Model file for the job. Use its own axes, mm. A direction names the side the tool comes from. Give positions to 0.01 mm unless a question says otherwise; leave off trailing zeros. Loops run counter-clockwise (first coordinate to the right, second up) from the corner with the lowest first, then second, coordinate; pieces in that order, holes last. Notation, with made-up numbers: (24.5, 25) - (28.5, 25) arc R16 cw to (28.5, 55) - close; hole circle Ø2 at (76, 51.25). An arc over 180 degrees is marked (long way). Use a Markdown table: item, result.
from build123d import *

# Parameters (mm, degrees)
F0_R        = 1.6
F1_DEPTH    = 1.5
F2_DEPTH    = 3.5
F3_T1_DEPTH = 1.5
F4_R        = 5


# Not quite as in the source:
# - a fillet or chamfer that OpenCascade refuses, or shapes differently, is made with other operations: its cross-section is extruded or revolved along the edge and cut away or added
# - a feature names something its author has since deleted; it is built from what else it names


with BuildPart() as f1:
    # F0 (on Top) → F1 (new body)
    with BuildSketch(Plane.XY):
        with BuildLine():
            Line((-18.9040250808, 5.7581766099), (-18.9040250808, 11.7581766099))
            Line((-18.9040250808, 11.7581766099), (-23.6040250808, 11.7581766099))
            Line((-23.6040250808, 11.7581766099), (-24.9040250808, 11.7581766099))
            Line((-24.9040250808, 11.7581766099), (-24.9040250808, -15.541421883))
            ThreePointArc((-24.9040250808, -15.541421883), (-22.6536235737, -17.7918233901), (-24.9040250808, -20.0422248973))
            Line((-24.9040250808, -20.0422248973), (-24.9040250808, -24.3918233901))
            ThreePointArc((-24.9040250808, -24.3918233901), (-21.9040250808, -21.3918233901), (-18.9040250808, -24.3918233901))
            Line((-18.9040250808, -24.3918233901), (-18.9040250808, -22.1418233901))
            Line((-18.9040250808, -22.1418233901), (-18.9040250808, -16.1418233901))
            Line((-18.9040250808, -16.1418233901), (-18.9040250808, 5.7581766099))
        make_face()
        with BuildLine():
            ThreePointArc((33.3459749192, 8.7581766099), (28.2246545756, 6.6368562663), (30.3459749192, 11.7581766099))
            Line((30.3459749192, 11.7581766099), (-17.6040250808, 11.7581766099))
            Line((-17.6040250808, 11.7581766099), (-18.9040250808, 11.7581766099))
            Line((-18.9040250808, 11.7581766099), (-18.9040250808, 5.7581766099))
            Line((-18.9040250808, 5.7581766099), (27.3459749192, 5.7581766099))
            Line((27.3459749192, 5.7581766099), (27.3459749192, -16.1418233901))
            Line((27.3459749192, -16.1418233901), (-18.9040250808, -16.1418233901))
            Line((-18.9040250808, -16.1418233901), (-18.9040250808, -22.1418233901))
            Line((-18.9040250808, -22.1418233901), (30.3459749192, -22.1418233901))
            ThreePointArc((30.3459749192, -22.1418233901), (28.2246545756, -17.0205030466), (33.3459749192, -19.1418233901))
            Line((33.3459749192, -19.1418233901), (33.3459749192, 8.7581766099))
        make_face()
        with BuildLine():
            ThreePointArc((-24.9040250808, -24.3918233901), (-21.9040250808, -27.3918233901), (-18.9040250808, -24.3918233901))
            ThreePointArc((-18.9040250808, -24.3918233901), (-21.9040250808, -21.3918233901), (-24.9040250808, -24.3918233901))
        make_face()
        with Locations((-21.9040250808, -24.3918233901)):
            Circle(F0_R, mode=Mode.SUBTRACT)
        with BuildLine():
            ThreePointArc((30.3459749192, -22.1418233901), (32.4672952628, -21.2631437337), (33.3459749192, -19.1418233901))
            ThreePointArc((33.3459749192, -19.1418233901), (28.2246545756, -17.0205030466), (30.3459749192, -22.1418233901))
        make_face()
        with Locations((30.3459749192, -19.1418233901)):
            Circle(F0_R, mode=Mode.SUBTRACT)
        with BuildLine():
            ThreePointArc((33.3459749192, 8.7581766099), (32.4672952628, 10.8794969534), (30.3459749192, 11.7581766099))
            ThreePointArc((30.3459749192, 11.7581766099), (28.2246545756, 6.6368562663), (33.3459749192, 8.7581766099))
        make_face()
        with Locations((30.3459749192, 8.7581766099)):
            Circle(F0_R, mode=Mode.SUBTRACT)
        with BuildLine():
            Line((-18.9040250808, 11.7581766099), (-17.6040250808, 11.7581766099))
            Line((-17.6040250808, 11.7581766099), (-17.6040250808, 24.3581766099))
            ThreePointArc((-17.6040250808, 24.3581766099), (-20.6040250808, 21.3581766099), (-23.6040250808, 24.3581766099))
            Line((-23.6040250808, 24.3581766099), (-23.6040250808, 11.7581766099))
            Line((-23.6040250808, 11.7581766099), (-18.9040250808, 11.7581766099))
        make_face()
        with BuildLine():
            ThreePointArc((-23.6040250808, 24.3581766099), (-20.6040250808, 21.3581766099), (-17.6040250808, 24.3581766099))
            ThreePointArc((-17.6040250808, 24.3581766099), (-20.6040250808, 27.3581766099), (-23.6040250808, 24.3581766099))
        make_face()
        with Locations((-20.6040250808, 24.3581766099)):
            Circle(F0_R, mode=Mode.SUBTRACT)
    extrude(amount=F1_DEPTH)

    # F0 (on Top) → F2 (join)
    with BuildSketch(Plane.XY):
        with BuildLine():
            ThreePointArc((-24.9040250808, -24.3918233901), (-21.9040250808, -27.3918233901), (-18.9040250808, -24.3918233901))
            ThreePointArc((-18.9040250808, -24.3918233901), (-21.9040250808, -21.3918233901), (-24.9040250808, -24.3918233901))
        make_face()
        with Locations((-21.9040250808, -24.3918233901)):
            Circle(F0_R, mode=Mode.SUBTRACT)
        with BuildLine():
            ThreePointArc((33.3459749192, 8.7581766099), (32.4672952628, 10.8794969534), (30.3459749192, 11.7581766099))
            ThreePointArc((30.3459749192, 11.7581766099), (28.2246545756, 6.6368562663), (33.3459749192, 8.7581766099))
        make_face()
        with Locations((30.3459749192, 8.7581766099)):
            Circle(F0_R, mode=Mode.SUBTRACT)
        with BuildLine():
            ThreePointArc((30.3459749192, -22.1418233901), (32.4672952628, -21.2631437337), (33.3459749192, -19.1418233901))
            ThreePointArc((33.3459749192, -19.1418233901), (28.2246545756, -17.0205030466), (30.3459749192, -22.1418233901))
        make_face()
        with Locations((30.3459749192, -19.1418233901)):
            Circle(F0_R, mode=Mode.SUBTRACT)
        with BuildLine():
            ThreePointArc((-23.6040250808, 24.3581766099), (-20.6040250808, 21.3581766099), (-17.6040250808, 24.3581766099))
            ThreePointArc((-17.6040250808, 24.3581766099), (-20.6040250808, 27.3581766099), (-23.6040250808, 24.3581766099))
        make_face()
        with Locations((-20.6040250808, 24.3581766099)):
            Circle(F0_R, mode=Mode.SUBTRACT)
    extrude(amount=F2_DEPTH)

    # F3: fillet of radius 5 on 7 edges, made by hand

    # F3_s2 → F3_t1 (join)
    with BuildSketch(Plane.XY):
        with BuildLine():
            ThreePointArc((-18.9040250808, 0.7581766099), (-17.4395589867, 4.2937105158), (-13.9040250808, 5.7581766099))
            Line((-13.9040250808, 5.7581766099), (-18.9040250808, 5.7581766099))
            Line((-18.9040250808, 5.7581766099), (-18.9040250808, 0.7581766099))
        make_face()
        with BuildLine():
            ThreePointArc((-18.9040250808, -11.1418233901), (-17.4395589867, -14.6773572961), (-13.9040250808, -16.1418233901))
            Line((-13.9040250808, -16.1418233901), (-18.9040250808, -16.1418233901))
            Line((-18.9040250808, -16.1418233901), (-18.9040250808, -11.1418233901))
        make_face()
        with BuildLine():
            ThreePointArc((22.3459749192, 5.7581766099), (25.8815088251, 4.2937105158), (27.3459749192, 0.7581766099))
            Line((27.3459749192, 0.7581766099), (27.3459749192, 5.7581766099))
            Line((27.3459749192, 5.7581766099), (22.3459749192, 5.7581766099))
        make_face()
        with BuildLine():
            ThreePointArc((22.3459749192, -16.1418233901), (25.8815088251, -14.6773572961), (27.3459749192, -11.1418233901))
            Line((27.3459749192, -11.1418233901), (27.3459749192, -16.1418233901))
            Line((27.3459749192, -16.1418233901), (22.3459749192, -16.1418233901))
        make_face()
        with BuildLine():
            ThreePointArc((-17.6040250808, 16.7581766099), (-16.1395589867, 13.2226427039), (-12.6040250808, 11.7581766099))
            Line((-12.6040250808, 11.7581766099), (-17.6040250808, 11.7581766099))
            Line((-17.6040250808, 11.7581766099), (-17.6040250808, 16.7581766099))
        make_face()
        with BuildLine():
            ThreePointArc((-24.9040250808, 11.7581766099), (-23.9403355543, 13.3184353163), (-23.6040250808, 15.121210954))
            Line((-23.6040250808, 15.121210954), (-23.6040250808, 11.7581766099))
            Line((-23.6040250808, 11.7581766099), (-24.9040250808, 11.7581766099))
        make_face()
        with BuildLine():
            ThreePointArc((-19.0868414806, -25.4230733901), (-17.2556452895, -23.0434243124), (-14.3915354801, -22.1418233901))
            Line((-14.3915354801, -22.1418233901), (-14.3915354801, -21.6418233901))
            Line((-14.3915354801, -21.6418233901), (-18.9040250808, -21.6418233901))
            Line((-18.9040250808, -21.6418233901), (-19.4040250808, -22.1418233901))
            ThreePointArc((-19.4040250808, -22.1418233901), (-19.4040250808, -24.3918233901), (-19.5563720806, -25.2511983901))
            Line((-19.5563720806, -25.2511983901), (-19.0868414806, -25.4230733901))
        make_face()
    extrude(amount=F3_T1_DEPTH)

    # F4
    f4_edges = [f1.edges().sort_by_distance(p)[0] for p in [
        (-24.904025, -15.541422, 0.75),
        (-24.904025, -20.042225, 0.75),
    ]]
    fillet(f4_edges, radius=F4_R)


solid = f1.part
(1) 3-axis set-ups, long thin cutter, end or side, ignore diameter. For faces 4 (the cylindrical face through (-24.488, -14.537, 0.76)), 5 (the flat face through (-17.604, 21, 1)), 6 (the flat face through (-23.604, 20, 1)), 7 (the flat face through (27.346, -5, 1)): which of +Z, -Z, +X, -X, +Y, -Y reach the whole face in a straight line?
Computed:
| item | result |
|---|---|
| face 4 | +Z, -Z, -X |
| face 5 | +Z, -Z, +X, +Y |
| face 6 | +Z, -Z, -X, +Y |
| face 7 | +Z, -Z |
(2) Slice it at A-A, the plane x = 2. Write the cut outline in (y, z), plus the area to 3 significant figures.
Computed:
| item | result |
|---|---|
| outline | (-22.14, 0) - (-16.14, 0) - (-16.14, 1.5) - (-22.14, 1.5) - close; (5.76, 0) - (11.76, 0) - (11.76, 1.5) - (5.76, 1.5) - close |
| area | 18.0 mm² |
(3) Slice it at C-C, the plane z = 0.75. Count the separate pieces of the cut face and the enclosed holes in it, plus the area to 3 significant figures.
Computed:
| item | result |
|---|---|
| separate pieces | 1 |
| enclosed holes | 5 |
| area | 1,060 mm² |
(4) Slice it at B-B, the plane y = -15.5. Write the cut outline in (x, z), plus the area to 3 significant figures.
Computed:
| item | result |
|---|---|
| outline | (-23.93, 0) - (-16.35, 0) - (-16.35, 1.5) - (-23.93, 1.5) - close; (24.8, 0) - (33.35, 0) - (33.35, 1.5) - (24.8, 1.5) - close |
| area | 24.2 mm² |
(5) Pin check, flat tips, straight feed: P1, Ø0.8, axis at y = 20, z = 1, coming from the -X side; P2, Ø0.8, axis at x = 9, z = 0.5, coming from the -Y side; P3, Ø1.6, axis at x = 3, z = 0.5, coming from the +Y side. Stop position of each tip, or through.
Computed:
| item | result |
|---|---|
| P1 | x = -23.6 |
| P2 | y = -22.14 |
| P3 | y = 11.76 |
(6) Drill centre lines: probe 1 along Y at (x, z) = (-7.5, 1); probe 2 along X at (y, z) = (-4, 1.4); probe 3 along Z at (x, y) = (-10.5, 10). Where is each one in solid material? Low to high. Write a range as [from, to].
Computed:
| item | result |
|---|---|
| probe 1 | [-22.14, -16.14], [5.76, 11.76] |
| probe 2 | [-24.9, -18.9], [27.35, 33.35] |
| probe 3 | [0, 1.5] |
(7) Mould opens along Y. For faces 1 (the cylindrical face through (-17.48, 4.25, 0.74)), 2 (the flat face through (-19, 23, 3.5)), 3 (the flat face through (8, -22.142, 1)) say: pulls with the +Y half, pulls with the -Y half, needs draft (parallel to the pull), parting line crosses it, or undercut.
Computed:
| item | result |
|---|---|
| face 1 | undercut |
| face 2 | needs draft |
| face 3 | pulls with the -Y half |
